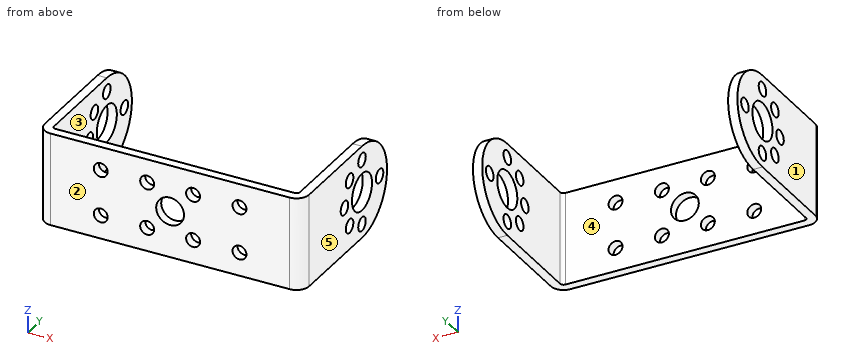
from build123d import *

# Parameters (mm, degrees)
SM_BASE_FLANGE_1_DEPTH = 20
EXTRUDE_1_DEPTH        = 2
EXTRUDE_START          = -2
EXTRUDE_2_DEPTH        = 2
SKETCH_8_R             = 4
SKETCH_8_R_2           = 1.5
CUT_EXTRUDE_1_DEPTH    = 65.618145883
SKETCH_9_R             = 3
SKETCH_9_R_2           = 1.5
CUT_EXTRUDE_2_DEPTH    = 2


# Sheet-metal steps are written as plain solids
with BuildPart() as part:
    # Sketch 1 → 基体-法兰1 (new body)
    with BuildSketch(Plane.XY):
        with BuildLine():
            Line((-12.079491004, 12.945691914), (-12.079491004, -8.117708086))
            ThreePointArc((-12.079491004, -8.117708086), (-11.863745859, -8.638562941), (-11.342891004, -8.854308086))
            Line((-11.342891004, -8.854308086), (40.183908996, -8.854308086))
            ThreePointArc((40.183908996, -8.854308086), (40.704763851, -8.638562941), (40.920508996, -8.117708086))
            Line((40.920508996, -8.117708086), (40.920508996, 12.945691914))
            Line((40.920508996, 12.945691914), (42.920508996, 12.945691914))
            Line((42.920508996, 12.945691914), (42.920508996, -8.117708086))
            ThreePointArc((42.920508996, -8.117708086), (42.118977413, -10.052776503), (40.183908996, -10.854308086))
            Line((40.183908996, -10.854308086), (-11.342891004, -10.854308086))
            ThreePointArc((-11.342891004, -10.854308086), (-13.277959422, -10.052776503), (-14.079491004, -8.117708086))
            Line((-14.079491004, -8.117708086), (-14.079491004, 12.945691914))
            Line((-14.079491004, 12.945691914), (-12.079491004, 12.945691914))
        make_face()
    extrude(amount=SM_BASE_FLANGE_1_DEPTH)

    # 草图6 → 凸台-拉伸1 (add)
    with BuildSketch(Plane.ZY.offset(14.079491004)):
        with BuildLine():
            Line((0, 12.945691914), (20, 12.945691914))
            ThreePointArc((20, 12.945691914), (10, 22.945691914), (0, 12.945691914))
        make_face()
    extrude(amount=-EXTRUDE_1_DEPTH)

    # 草图7 → 凸台-拉伸2 (add)
    with BuildSketch(Plane(origin=(42.920508996, 0, 0), x_dir=(0, 0, -1), z_dir=(1, 0, 0)).offset(EXTRUDE_START)):
        with BuildLine():
            Line((-20, 12.945691914), (0, 12.945691914))
            ThreePointArc((0, 12.945691914), (-10, 22.945691914), (-20, 12.945691914))
        make_face()
    extrude(amount=EXTRUDE_2_DEPTH)

    # 草图8 → 切除-拉伸1 (cut, through all)
    with BuildSketch(Plane.ZY.offset(14.079491004)):
        with Locations((10, 12.945691914)):
            Circle(SKETCH_8_R)
        with Locations((10, 19.945691914)):
            Circle(SKETCH_8_R_2)
        with Locations((17, 12.945691914)):
            Circle(SKETCH_8_R_2)
        with Locations((14.949747468, 7.995944446)):
            Circle(SKETCH_8_R_2)
        with Locations((10, 5.945691914)):
            Circle(SKETCH_8_R_2)
        with Locations((5.050252532, 7.995944446)):
            Circle(SKETCH_8_R_2)
        with Locations((3, 12.945691914)):
            Circle(SKETCH_8_R_2)
    extrude(amount=-CUT_EXTRUDE_1_DEPTH, mode=Mode.SUBTRACT)

    # 草图9 → 切除-拉伸2 (cut)
    with BuildSketch(Plane(origin=(0, -10.854308086, 0), x_dir=(-1, 0, 0), z_dir=(0, -1, 0))):
        with Locations(Location((-14.420508996, -10, 0), (0, 0, 90))):
            Circle(SKETCH_9_R)
        with Locations(Location((-29.370256464, -5.050252532, 0), (0, 0, 90))):
            Circle(SKETCH_9_R_2)
        with Locations(Location((-19.370256464, -5.050252532, 0), (0, 0, 90))):
            Circle(SKETCH_9_R_2)
        with Locations(Location((-9.470761527, -5.050252532, 0), (0, 0, 90))):
            Circle(SKETCH_9_R_2)
        with Locations(Location((-19.370256464, -14.949747468, 0), (0, 0, 90))):
            Circle(SKETCH_9_R_2)
        with Locations(Location((-9.470761527, -14.949747468, 0), (0, 0, 90))):
            Circle(SKETCH_9_R_2)
        with Locations(Location((-29.370256464, -14.949747468, 0), (0, 0, 90))):
            Circle(SKETCH_9_R_2)
        with Locations(Location((0.529238473, -5.050252532, 0), (0, 0, 90))):
            Circle(SKETCH_9_R_2)
        with Locations(Location((0.529238473, -14.949747468, 0), (0, 0, 90))):
            Circle(SKETCH_9_R_2)
    extrude(amount=-CUT_EXTRUDE_2_DEPTH, mode=Mode.SUBTRACT)


solid = part.part
Part model, mm, in its own coordinate system. Face numbers are marked on the shaded views. A direction names the side the tool comes from. Round coordinates to 2 decimals unless told otherwise and drop trailing zeros. Loops run counter-clockwise (first coordinate to the right, second up) from the corner with the lowest first, then second, coordinate; pieces in that order, holes last. Notation, with made-up numbers: (34, -23.5) - (53, -23.5) arc R9 ccw to (53, -19.5) - close; hole circle Ø7 at (-14.75, 20.5). An arc over 180 degrees is marked (long way). Answer as a JSON object with one key per item and string values.
Item 1: Band-saw the part on A-A on y = -6. List the corners of the cut face in (x, z), plus the area to 3 significant figures.
Output:
{"outline": "(-14.08, 0) - (-12.08, 0) - (-12.08, 20) - (-14.08, 20) - close; (40.92, 0) - (42.92, 0) - (42.92, 20) - (40.92, 20) - close", "area": "80.0 mm2"}
Item 2: Tool access for the marked faces 4 and 5: list every direction of +Z, -Z, +X, -X, +Y, -Y with a clear straight run to the whole face (end or side of a thin tool).
Output:
{"face 4": "+Z, -Z, +Y", "face 5": "+Z, -Z, +X, +Y, -Y"}
Item 3: Band-saw the part on C-C on y = 19. List the corners of the cut face in (x, z), plus the area to 3 significant figures.
Output:
{"outline": "(-14.08, 2.04) - (-12.08, 2.04) - (-12.08, 8.84) - (-14.08, 8.84) - close; (-14.08, 11.16) - (-12.08, 11.16) - (-12.08, 17.96) - (-14.08, 17.96) - close; (40.92, 2.04) - (42.92, 2.04) - (42.92, 8.84) - (40.92, 8.84) - close; (40.92, 11.16) - (42.92, 11.16) - (42.92, 17.96) - (40.92, 17.96) - close", "area": "54.4 mm2"}
Item 4: Band-saw the part on D-D on z = 10. State how many separate pieces and enclosed holes the cut face has, plus the area to 3 significant figures.
Output:
{"separate pieces": "8", "enclosed holes": "0", "area": "170 mm2"}
Item 5: Pull direction X, two halves, no side cores. Call the marked faces 1, 2 and 3: pulls with the +X half, pulls with the -X half, needs draft (parallel to the pull), parting line crosses it, or undercut.
Output:
{"face 1": "pulls with the -X half", "face 2": "needs draft", "face 3": "undercut"}
Item 6: Band-saw the part on B-B on z = 2.25. List the corners of the cut face in (x, y), plus the area to 3 significant figures.
Output:
{"outline": "(-14.08, -8.12) arc R2.74 ccw to (-11.34, -10.85) - (40.18, -10.85) arc R2.74 ccw to (42.92, -8.12) - (42.92, 11.65) - (40.92, 11.65) - (40.92, -8.12) arc R0.74 cw to (40.18, -8.85) - (-11.34, -8.85) arc R0.74 cw to (-12.08, -8.12) - (-12.08, 11.65) - (-14.08, 11.65) - close; (-14.08, 14.24) - (-12.08, 14.24) - (-12.08, 19.27) - (-14.08, 19.27) - close; (40.92, 14.24) - (42.92, 14.24) - (42.92, 19.27) - (40.92, 19.27) - close", "area": "213 mm2"}
Item 7: Wall check: L1, parallel to X at y = -6, z = 15; L2, parallel to Y at x = 9, z = 18; L3, parallel to Y at x = -13.2, z = 10. Give the ranges that are in metal, low to high.
Output:
{"L1": "-14.08 to -12.08, 40.92 to 42.92", "L2": "-10.85 to -8.85", "L3": "-10.13 to 4.45, 7.45 to 8.95, 16.95 to 18.45, 21.45 to 22.95"}
Item 8: Pin check, flat tip, straight feed: pin 1 (4 mm diameter, centred on x = -0.53, z = 14.95, fed in from +Y). Stop position of the tip, or through.
Output:
{"pin 1": "y = -8.85"}
